The model under review builds one solid part; all positions refer to its coordinate system, in mm. A direction names the side the tool comes from. Give positions to 0.01 mm unless a question says otherwise; leave off trailing zeros. Loops run counter-clockwise (first coordinate to the right, second up) from the corner with the lowest first, then second, coordinate; pieces in that order, holes last. Notation, with made-up numbers: M 15.25,86.5 L 34.25,86.5 A13 ccw 34.25,105.5 Z; hole C -10.5,-7.75 d7. An arc over 180 degrees is marked long. One line per item, written item: value. Start each with the question number.
Q1. Mouldability with a two-part tool opening along Z and no side actions: class faces 6 (the face through (7, 16, 10)), 7 (the face through (52, 11, 0)), 8 (the face through (25.362, 2.971, 5.043)), 9 (the face through (15, 19, 13)) as released by +Z, released by -Z, zero draft, split by the parting line, or undercut.
Q2. We need section C-C on y = 3.25. Write out the cut boundary in (x, z).
Q3. For faces 1 (the face through (90, 19, 13)), 2 (the face through (25, 22, 8)), 3 (the face through (41.5, 20, 14)), 4 (the face through (52, 9, 16)), 5 (the face through (63.5, 24, 3)), list the 3-axis set-ups (+Z, -Z, +X, -X, +Y, -Y) from which the entire face can be reached by the end or side of a thin tool; tool diameter is ignored.
Q4. We need section D-D on x = 93.5. Write out the cut boundary in (y, z), plus the area to 3 significant figures.
Q5. We need section B-B on x = 75. Write out the cut boundary in (y, z) (3 decimals).
Q6. For pin 1 (8.5 mm diameter, centred on x = 30, z = 8, fed in from +Y); pin 2 (2 mm diameter, centred on y = 19, z = 13, fed in from -X); pin 3 (7.5 mm diameter, centred on y = 18.5, z = 13, fed in from +X); pin 4 (5.5 mm diameter, centred on x = 75.5, z = 8, fed in from -Y), all flat-tipped, find the tip position at first contact; note any pin that passes through.
Q7. We need section A-A on z = 8. Give the number of separate pieces and of enclosed holes in the cut face, plus the area to 3 significant figures.
Q8. To check wall thickness, follow line 1 along X through (y, z) = (17.25, 8); line 2 along X through (y, z) = (1.3, 8); line 3 along Z through (x, y) = (30, 2.2). State the ranges of each line that lie inside material, in increasing order. Write a range as from..to.
```python
from build123d import *

# Parameters (mm, degrees)
CROQUIS1_W                                   = 105
CROQUIS1_H                                   = 22
SALIENTE_EXTRUIR1_DEPTH                      = 16
CORTAR_EXTRUIR2_DEPTH                        = 15
CORTAR_EXTRUIR3_START                        = -105
CORTAR_EXTRUIR3_DEPTH                        = 15
CROQUIS3_W                                   = 22
CROQUIS3_H                                   = 14
CORTAR_EXTRUIR4_DEPTH                        = 109.466584716
SALIENTE_EXTRUIR3_DEPTH                      = 22
CROQUIS5_R                                   = 7.45
CORTAR_EXTRUIR6_DEPTH                        = 15
REFRENTADO_PARA_TORNILLO_TAP_N_CON_C_2_COUNT = 2
REFRENTADO_PARA_TORNILLO_TAP_N_CON_C_2_PITCH = 45


with BuildPart() as part:
    # Croquis1 → Saliente-Extruir1 (new body)
    with BuildSketch(Plane.XY):
        with Locations((52.5, 11)):
            Rectangle(CROQUIS1_W, CROQUIS1_H)
    extrude(amount=SALIENTE_EXTRUIR1_DEPTH)

    # Croquis2 → Cortar-Extruir2 (cut)
    with BuildSketch(Plane(origin=(105, 0, 0), x_dir=(0, 0, -1), z_dir=(1, 0, 0))):
        Polygon((-16, 10), (-16, 22), (-4, 22), align=None)
    extrude(amount=-CORTAR_EXTRUIR2_DEPTH, mode=Mode.SUBTRACT)

    # Croquis2<2> → Cortar-Extruir3 (cut)
    with BuildSketch(Plane(origin=(105, 0, 0), x_dir=(0, 0, -1), z_dir=(1, 0, 0)).offset(CORTAR_EXTRUIR3_START)):
        Polygon((-16, 10), (-16, 22), (-4, 22), align=None)
    extrude(amount=CORTAR_EXTRUIR3_DEPTH, mode=Mode.SUBTRACT)

    # Croquis3 → Cortar-Extruir4 (cut, through all)
    with BuildSketch(Plane.XY.offset(16)):
        with Locations((52.5, 22)):
            Rectangle(CROQUIS3_W, CROQUIS3_H)
    extrude(amount=-CORTAR_EXTRUIR4_DEPTH, mode=Mode.SUBTRACT)

    # Croquis4 → Saliente-Extruir3 (add)
    with BuildSketch(Plane(origin=(41.5, 0, 0), x_dir=(0, 0, -1), z_dir=(1, 0, 0))):
        Polygon((-16, 15), (-3, 28), (0, 28), (0, 15), align=None)
    extrude(amount=SALIENTE_EXTRUIR3_DEPTH)

    # Croquis5 → Cortar-Extruir6 (cut)
    with BuildSketch(Plane(origin=(0, 0, 0), x_dir=(-1, 0, 0), z_dir=(0, 0, -1))):
        with Locations((-52.5, 32)):
            Circle(CROQUIS5_R)
    extrude(amount=-CORTAR_EXTRUIR6_DEPTH, mode=Mode.SUBTRACT)

    # Croquis9 → Refrentado para tornillo tapón con cabeza de clavija de M61 (revolve, cut)
    with BuildSketch(Plane(origin=(30, 0, 8), x_dir=(0, 0, -1), z_dir=(1, 0, 0))):
        Polygon((0, 0), (0, 28), (3.3, 28), (3.3, 6), (5.5, 6), (5.5, 0.025), (5.525, 0), align=None)
    refrentado_para_tornillo_tap_n_con_cabez = revolve(axis=Axis((30, -6.35, 8), (0, 1, 0)), mode=Mode.SUBTRACT)

    # Refrentado para tornillo tap_n con c 2: Refrentado para tornillo tapón con cabeza de clavija de M61 ×2
    with Locations(*[(i * REFRENTADO_PARA_TORNILLO_TAP_N_CON_C_2_PITCH, 0, 0) for i in range(1, REFRENTADO_PARA_TORNILLO_TAP_N_CON_C_2_COUNT)]):
        add(refrentado_para_tornillo_tap_n_con_cabez, mode=Mode.SUBTRACT)


solid = part.part
```
Solved:
1. face 6: released by +Z
1. face 7: released by -Z
1. face 8: undercut
1. face 9: zero draft
2. outline: M 0,0 L 105,0 L 105,16 L 0,16 Z; hole C 30,8 d11; hole C 75,8 d11
3. face 1: +Z, +X, +Y
3. face 2: +Z, -Z, -X, +Y
3. face 3: +Z, +Y
3. face 4: +Z, +X, -X, +Y, -Y
3. face 5: +Z, -Z, +X, +Y
4. outline: M 0,0 L 22,0 L 22,4 L 10,16 L 0,16 Z
4. area: 280 mm2
5. outline: M 0,0 L 22,0 L 22,4.7 L 6,4.7 L 6,2.5 L 0.025,2.5 L 0,2.475 Z; M 0,13.525 L 0.025,13.5 L 6,13.5 L 6,11.3 L 22,11.3 L 22,16 L 0,16 Z
6. pin 1: y = 22
6. pin 2: x = 15
6. pin 3: x = 90
6. pin 4: through
7. separate pieces: 3
7. enclosed holes: 0
7. area: 1,870 mm2
8. line 1: 0..26.7, 33.3..71.7, 78.3..105
8. line 2: 0..24.5, 35.5..69.5, 80.5..105
8. line 3: 0..2.5, 13.5..16
